Here's the drawing with two shaded views (mm, measured from the low corner). I have some questions. Give positions to 0.01 mm unless a question says otherwise; leave off trailing zeros. Write each loop counter-clockwise with the first axis right and the second up, starting at its lowest first coordinate (ties: lowest second). Pieces come first, ordered by that corner, then holes. Notation, with made-up numbers: (13.25, -24.75) - (53.25, -24.75) arc R20 ccw to (53.25, 6.25) - close; hole circle Ø1 at (25, 78.25). An arc over 180 degrees is marked (long way). Write item = value, one per line.
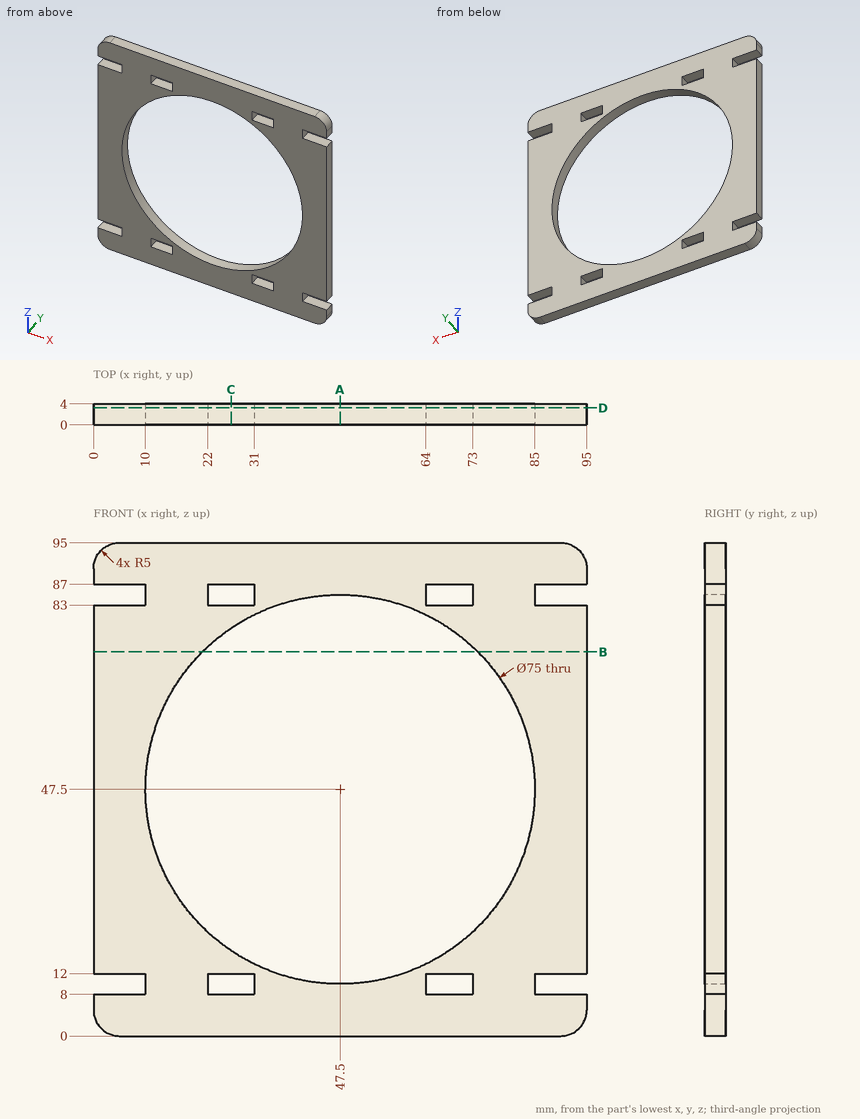
1. I need wall thicknesses on line 1 (X direction, y = 1.1, z = 47.5); line 2 (Z direction, x = 25.5, y = 3.75); line 3 (Z direction, x = 61, y = 3.8). Which ranges of each line are inside material? Lowest first, please.
Filled sheet:
line_1 = 0 to 10, 85 to 95
line_2 = 0 to 8, 12 to 17.13, 77.87 to 83, 87 to 95
line_3 = 0 to 12.51, 82.49 to 95
2. If we section it at B-B, the plane z = 74: Please give me the cut outline in (x, y).
Filled sheet:
outline = (0, 0) - (20.97, 0) - (20.97, 4) - (0, 4) - close; (74.03, 0) - (95, 0) - (95, 4) - (74.03, 4) - close
3. For pin 1 (2 mm diameter, centred on y = 2.5, z = 84.5, fed in from -X); pin 2 (2 mm diameter, centred on y = 3, z = 10.5, fed in from +X); pin 3 (1.2 mm diameter, centred on x = 3.5, y = 1.5, fed in from -Z), each with a flat end and sliding along its axis, tell me the tip position at first contact or that it passes through.
Filled sheet:
pin_1 = 10
pin_2 = 85
pin_3 = 0.08
4. If we section it at A-A, the plane x = 47.5: Please give me the cut outline in (y, z), and give its area (3 significant figures).
Filled sheet:
outline = (0, 0) - (4, 0) - (4, 10) - (0, 10) - close; (0, 85) - (4, 85) - (4, 95) - (0, 95) - close
area = 80.0 mm2
5. If we section it at C-C, the plane x = 26.5: Please give me the cut outline in (y, z).
Filled sheet:
outline = (0, 0) - (4, 0) - (4, 8) - (0, 8) - close; (0, 12) - (4, 12) - (4, 16.43) - (0, 16.43) - close; (0, 78.57) - (4, 78.57) - (4, 83) - (0, 83) - close; (0, 87) - (4, 87) - (4, 95) - (0, 95) - close
6. If we section it at D-D, the plane y = 3.25: Count the separate pieces of the cut face and the enclosed holes in it, and give its area (3 significant figures).
Filled sheet:
separate_pieces = 1
enclosed_holes = 5
area = 4,280 mm2
